Check sheet for the modelled part. Datum: model origin and axes. Units: mm. A direction names the side the tool comes from. Give positions to 0.01 mm unless a question says otherwise; leave off trailing zeros. Loops run counter-clockwise (first coordinate to the right, second up) from the corner with the lowest first, then second, coordinate; pieces in that order, holes last. Notation, with made-up numbers: (20.5, 26) - (74.5, 26) arc R28 cw to (74.5, 48) - close; hole circle Ø4 at (66.25, -6.75). An arc over 180 degrees is marked (long way). Use CSV: the item, a comma, the result in double quotes.
from build123d import *

# Parameters (mm, degrees)
SKETCH2_W           = 50.8
SKETCH2_H           = 25.4
BOSS_EXTRUDE2_DEPTH = 1.999996
SKETCH2_4_W         = 46.5836
SKETCH2_4_H         = 21.1836
BOSS_EXTRUDE3_DEPTH = 25.4
FILLET3_R           = 0.79375
SKETCH3_R           = 2.54
CUT_EXTRUDE1_DEPTH  = 49.6918
SKETCH4_R           = 2.54
CUT_EXTRUDE2_DEPTH  = 24.2918
SKETCH5_W           = 46.5836
SKETCH5_H           = 18.796
CUT_EXTRUDE3_DEPTH  = 6.35
FILLET4_R           = 0.762


with BuildPart() as part:
    # Sketch2 → Boss-Extrude2 (new body)
    with BuildSketch(Plane(origin=(0, 0, 0), x_dir=(1, 0, 0), z_dir=(0, 1, 0))):
        with Locations((25.4, 12.7)):
            Rectangle(SKETCH2_W, SKETCH2_H)
    extrude(amount=BOSS_EXTRUDE2_DEPTH)

    # Sketch2<4> → Boss-Extrude3 (add)
    with BuildSketch(Plane(origin=(0, 0, 0), x_dir=(1, 0, 0), z_dir=(0, 1, 0))):
        with Locations((25.4, 12.7)):
            Rectangle(SKETCH2_4_W, SKETCH2_4_H)
    extrude(amount=-BOSS_EXTRUDE3_DEPTH)

    # Fillet3
    fillet3_edges = [part.edges().sort_by_distance(p)[0] for p in [
        (2.1082, -12.7, -2.1082),
        (2.1082, -12.7, -23.2918),
        (48.6918, -12.7, -23.2918),
        (48.6918, -12.7, -2.1082),
    ]]
    fillet(fillet3_edges, radius=FILLET3_R)

    # Sketch3 → Cut-Extrude1 (cut, through all)
    with BuildSketch(Plane(origin=(48.6918, 0, 0), x_dir=(0, 0, -1), z_dir=(1, 0, 0))):
        with Locations((12.7, -12.7)):
            Circle(SKETCH3_R)
    extrude(amount=-CUT_EXTRUDE1_DEPTH, mode=Mode.SUBTRACT)

    # Sketch4 → Cut-Extrude2 (cut, through all)
    with BuildSketch(Plane(origin=(0, 0, -23.2918), x_dir=(-1, 0, 0), z_dir=(0, 0, -1))):
        with Locations((-25.4, -12.7)):
            Circle(SKETCH4_R)
        with Locations((-38.1, -12.7)):
            Circle(SKETCH4_R)
        with Locations((-12.7, -12.7)):
            Circle(SKETCH4_R)
    extrude(amount=-CUT_EXTRUDE2_DEPTH, mode=Mode.SUBTRACT)

    # Sketch5 → Cut-Extrude3 (cut)
    with BuildSketch(Plane(origin=(0, 0, -23.2918), x_dir=(-1, 0, 0), z_dir=(0, 0, -1))):
        with Locations((-25.4, -16.002)):
            Rectangle(SKETCH5_W, SKETCH5_H)
    extrude(amount=-CUT_EXTRUDE3_DEPTH, mode=Mode.SUBTRACT)

    # Fillet4
    fillet4_edges = [part.edges().sort_by_distance(p)[0] for p in [
        (2.1082, -16.002, -16.9418),
        (48.6918, -16.002, -16.9418),
    ]]
    fillet(fillet4_edges, radius=FILLET4_R)


solid = part.part
1. Scan lines: line 1 along X through (y, z) = (-12.7, -8); line 2 along Y through (x, z) = (6.5, -12.7); line 3 along Z through (x, y) = (46.75, -12.7). Record each from-to range of solid material in increasing order.
Completed:
line 1,"x = 2.11 to 10.16, 15.24 to 22.86, 27.94 to 35.56, 40.64 to 48.69"
line 2,"y = -25.4 to -15.24, -10.16 to 2"
line 3,"z = -16.94 to -15.24, -10.16 to -2.11"
2. Go/stop test with flat-tipped pins: pin 1 Ø6 at (x, y) = (37.5, -20) entering from +Z; pin 2 Ø10 at (y, z) = (-13, -11) entering from +X; pin 3 Ø3 at (x, y) = (7.5, -15.5) entering from -Z; pin 4 Ø8 at (x, z) = (29.5, -18.5) entering from -Y. Record where each tip stops, or that it passes through.
Completed:
pin 1,"stops at z = -2.11"
pin 2,"stops at x = 48.69"
pin 3,"stops at z = -16.94"
pin 4,"stops at y = -25.4"
3. Sectioned sample at C-C, the plane y = -6. Record the boundary of the cut face in (x, z), and give its area (3 significant figures).
Completed:
outline,"(2.11, -22.5) arc R0.79 ccw to (2.9, -23.29) - (47.9, -23.29) arc R0.79 ccw to (48.69, -22.5) - (48.69, -2.9) arc R0.79 ccw to (47.9, -2.11) - (2.9, -2.11) arc R0.79 ccw to (2.11, -2.9) - close"
area,"986 mm²"
4. Sectioned sample at D-D, the plane y = -14.5. State how many separate pieces and enclosed holes the cut face has, and give its area (3 significant figures).
Completed:
separate pieces,"8"
enclosed holes,"0"
area,"403 mm²"
5. Sectioned sample at A-A, the plane z = -7.5. Record the boundary of the cut face in (x, y).
Completed:
outline,"(0, 0) - (2.11, 0) - (2.11, -25.4) - (48.69, -25.4) - (48.69, 0) - (50.8, 0) - (50.8, 2) - (0, 2) - close; hole circle Ø5.08 at (12.7, -12.7); hole circle Ø5.08 at (25.4, -12.7); hole circle Ø5.08 at (38.1, -12.7)"
6. Set-up check for faces 4 (the face through (2.108, -10, -10)), 5 (the face through (48.692, -10, -10)), 6 (the face through (25, -3, -23.292)), 7 (the face through (44.647, -13.673, -15.046)), 8 (the face through (23, 0, -1)): record each of +Z, -Z, +X, -X, +Y, -Y from which the full face is reachable in a straight line by a thin tool's end or side.
Completed:
face 4,"+Z, -Z, -X, -Y"
face 5,"+Z, -Z, +X, -Y"
face 6,"-Z, +X, -X, -Y"
face 7,"+X, -X"
face 8,"-Y"
7. Release check for a two-part mould opening along Y. For faces 1 (the face through (25, 1, -25.4)), 2 (the face through (19.139, -12.588, -10.162)), 3 (the face through (26, -6.604, -21)) record: released by +Y, released by -Y, zero draft, split by the parting line, or undercut.
Completed:
face 1,"zero draft"
face 2,"undercut"
face 3,"released by -Y"
8. Sectioned sample at B-B, the plane x = 33. Record the boundary of the cut face in (y, z), and give its area (3 significant figures).
Completed:
outline,"(-25.4, -16.94) - (-6.6, -16.94) - (-6.6, -23.29) - (0, -23.29) - (0, -25.4) - (2, -25.4) - (2, 0) - (0, 0) - (0, -2.11) - (-25.4, -2.11) - close; hole circle Ø5.08 at (-12.7, -12.7)"
area,"449 mm²"
